from build123d import *

# Parameters (mm, degrees)
F0_W     = 31
F0_H     = 57
F1_DEPTH = 15
F2_R     = 5
F3_W     = 11.5
F3_H     = 54
F4_DEPTH = 10


with BuildPart() as f1:
    # F0 (on Top) → F1 (new body)
    with BuildSketch(Plane.XY):
        Rectangle(F0_W, F0_H)
    extrude(amount=F1_DEPTH)

    # F2
    f2_edges = [f1.edges().sort_by_distance(p)[0] for p in [
        (15.5, 0, 15),
        (-15.5, 0, 15),
    ]]
    fillet(f2_edges, radius=F2_R)

    # F3 (on face) → F4 (cut)
    with BuildSketch(Plane.XY.offset(15)):
        with Locations((7.75, 0.5)):
            Rectangle(F3_W, F3_H)
        with Locations((-7.75, 0.5)):
            Rectangle(F3_W, F3_H)
    extrude(amount=-F4_DEPTH, mode=Mode.SUBTRACT)


solid = f1.part
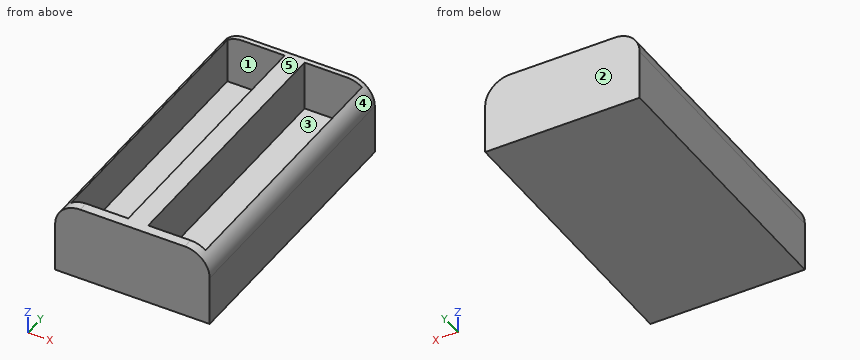
Source: CAD feature listing. Evaluate the final solid. Frame: model axes, mm. Face numbers are marked on the shaded views. A direction names the side the tool comes from. Give positions to 0.01 mm unless a question says otherwise; leave off trailing zeros. Order: outer loops, then holes, each group sorted by start corner. A loop starts at its lowest first (then second) coordinate and runs counter-clockwise, first axis right, second up. Notation, with made-up numbers: (67, 53) -> (73, 53) arc R21 ccw to (73, 88) -> close; hole circle Ø2 at (41, 47.5). An arc over 180 degrees is marked (long way). Write item = value, one per line.
Item 1: Contact query for flat-ended pins moving along their axis: pin 1 (1 mm diameter, centred on y = -6, z = 11, fed in from +X); pin 2 (3.5 mm diameter, centred on x = -7.5, y = -12.5, fed in from +Z). Output: stop coordinate, or through.
Check result:
pin_1 = 15.47
pin_2 = 5
Item 2: Section query B-B (x = 5). Output: boundary loops of the cut face in (y, z), then the cut area to 3 significant figures.
Check result:
outline = (-28.5, 0) -> (28.5, 0) -> (28.5, 15) -> (27.5, 15) -> (27.5, 5) -> (-26.5, 5) -> (-26.5, 15) -> (-28.5, 15) -> close
area = 315 mm²
Item 3: Section query D-D (z = 13). Output: boundary loops of the cut face in (x, y).
Check result:
outline = (-14.5, -28.5) -> (14.5, -28.5) -> (14.5, 28.5) -> (-14.5, 28.5) -> close; hole (-13.5, -26.5) -> (-2, -26.5) -> (-2, 27.5) -> (-13.5, 27.5) -> close; hole (2, -26.5) -> (13.5, -26.5) -> (13.5, 27.5) -> (2, 27.5) -> close
Item 4: Section query C-C (y = 18). Output: boundary loops of the cut face in (x, z).
Check result:
outline = (-15.5, 0) -> (15.5, 0) -> (15.5, 10) arc R5 ccw to (13.5, 14) -> (13.5, 5) -> (2, 5) -> (2, 15) -> (-2, 15) -> (-2, 5) -> (-13.5, 5) -> (-13.5, 14) arc R5 ccw to (-15.5, 10) -> close
Item 5: Ray query, probe 1 along X at (y, z) = (-5, 7); probe 2 along Y at (x, z) = (10, 14); probe 3 along X at (y, z) = (-25.5, 12). Return the intervals inside material, ascending.
Check result:
probe_1 = -15.5 to -13.5, -2 to 2, 13.5 to 15.5
probe_2 = -28.5 to -26.5, 27.5 to 28.5
probe_3 = -15.08 to -13.5, -2 to 2, 13.5 to 15.08
Item 6: Section query A-A (z = 7). Output: boundary loops of the cut face in (x, y).
Check result:
outline = (-15.5, -28.5) -> (15.5, -28.5) -> (15.5, 28.5) -> (-15.5, 28.5) -> close; hole (-13.5, -26.5) -> (-2, -26.5) -> (-2, 27.5) -> (-13.5, 27.5) -> close; hole (2, -26.5) -> (13.5, -26.5) -> (13.5, 27.5) -> (2, 27.5) -> close
Item 7: Set-up query: the marked faces 1 and 2. Return all of +Z, -Z, +X, -X, +Y, -Y with unobstructed straight access to the full face (end or side cutting, diameter ignored); none if empty.
Check result:
face_1 = +Z
face_2 = +Z, -Z, +X, -X, +Y
Item 8: Mould query, pull axis X, two halves, no side actions, for the marked faces 3, 4 and 5. Classes: +X half, -X half, draft (parallel to the pull), parting line (faces both ways), or undercut.
Check result:
face_3 = undercut
face_4 = +X half
face_5 = draft
